Part print with two shaded views. Sizes in mm from the minimum x, y, z corner. A direction names the side the tool comes from. Round coordinates to 2 decimals unless told otherwise and drop trailing zeros. Loops run counter-clockwise (first coordinate to the right, second up) from the corner with the lowest first, then second, coordinate; pieces in that order, holes last.
(1) Probe probe 1 along Y at (x, z) = (2.45, 22); probe 2 along X at (y, z) = (16.75, 12.5). List the from-to ranges inside material, lowest first.
(2) Tool access for the marked faces 1, 2 and 3: list every direction of +Z, -Z, +X, -X, +Y, -Y with a clear straight run to the whole face (end or side of a thin tool).
(3) Cut at B-B on y = 7. List the corners of the cut face in (x, z), then the cut area to 3 significant figures.
(4) Flat gauge pins, fed straight in: pin 1 (3 mm diameter, centred on y = 11.5, z = 22, fed in from +X); pin 2 (5 mm diameter, centred on x = 11.8, z = 21.25, fed in from +Y); pin 3 (4 mm diameter, centred on y = 3, z = 10, fed in from +X). Where does each tip first touch, or does it go through?
(5) Cut at C-C on z = 3.75. List the corners of the cut face in (x, y).
(6) Cut at A-A on x = 40. List the corners of the cut face in (y, z).
(7) Cut at D-D on y = 4.25. List the corners of the cut face in (x, z).
(8) Mould opens along Z. For the marked faces 4, 5 and 6 say: +Z half, -Z half, draft (parallel to the pull), parting line (faces both ways), or undercut.
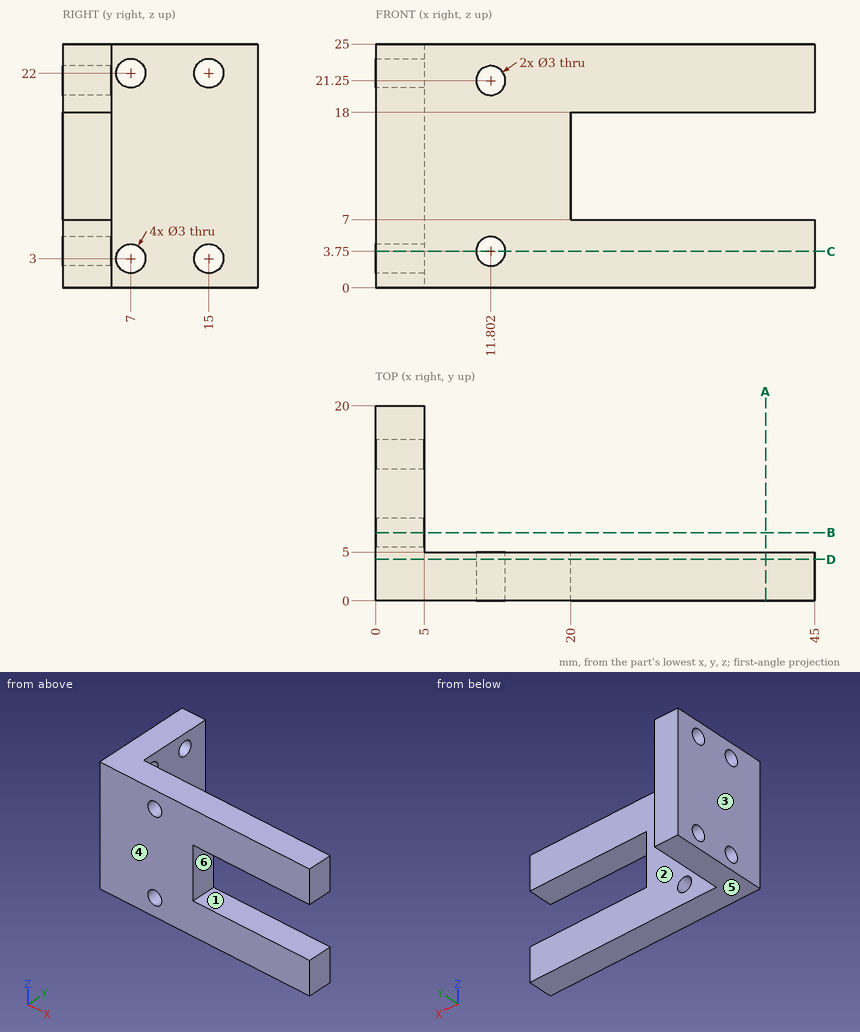
Final values:
1. probe 1: y = 0 to 5.5, 8.5 to 13.5, 16.5 to 20
1. probe 2: x = 0 to 5
2. face 1: +X, +Y, -Y
2. face 2: +Z, -Z, +X, +Y
2. face 3: +Z, -Z, -X, +Y, -Y
3. outline: (0, 0) - (5, 0) - (5, 1.5) - (0, 1.5) - close; (0, 4.5) - (5, 4.5) - (5, 20.5) - (0, 20.5) - close; (0, 23.5) - (5, 23.5) - (5, 25) - (0, 25) - close
3. area: 95.0 mm2
4. pin 1: stops at x = 5
4. pin 2: stops at y = 5
4. pin 3: stops at x = 20
5. outline: (0, 0) - (10.3, 0) - (10.3, 5) - (5, 5) - (5, 5.7) - (0, 5.7) - close; (0, 8.3) - (5, 8.3) - (5, 13.7) - (0, 13.7) - close; (0, 16.3) - (5, 16.3) - (5, 20) - (0, 20) - close; (13.3, 0) - (45, 0) - (45, 5) - (13.3, 5) - close
6. outline: (0, 0) - (5, 0) - (5, 7) - (0, 7) - close; (0, 18) - (5, 18) - (5, 25) - (0, 25) - close
7. outline: (0, 0) - (45, 0) - (45, 7) - (20, 7) - (20, 18) - (45, 18) - (45, 25) - (0, 25) - close; hole circle Ø3 at (11.8, 3.75); hole circle Ø3 at (11.8, 21.25)
8. face 4: draft
8. face 5: -Z half
8. face 6: undercut
